```python
from build123d import *

# Parameters (mm, degrees)
BOSS_EXTRUDE1_DEPTH = 3
SKETCH2_R           = 1.5
CUT_EXTRUDE1_DEPTH  = 302.770194022
SKETCH3_R           = 1.5
CUT_EXTRUDE2_DEPTH  = 302.770194022
LPATTERN1_COUNT     = 6
LPATTERN1_PITCH     = 15


with BuildPart() as part:
    # Sketch1 → Boss-Extrude1 (new body)
    with BuildSketch(Plane(origin=(0, 0, 0), x_dir=(1, 0, 0), z_dir=(0, 1, 0))):
        Polygon((32.5, 300), (-32.5, 300), (-32.5, 270), (-15, 270), (-15, 90), (-21, 90), (-21, 0), (21, 0), (21, 90), (15, 90), (15, 270), (32.5, 270), align=None)
    extrude(amount=BOSS_EXTRUDE1_DEPTH)

    # Sketch2 → Cut-Extrude1 (cut, symmetric)
    with BuildSketch(Plane(origin=(0, 3, 0), x_dir=(1, 0, 0), z_dir=(0, 1, 0))):
        with Locations(Location((-28, 295.85, 0), (0, 0, 270))):
            Circle(SKETCH2_R)
        with Locations(Location((-7, 295.85, 0), (0, 0, 270))):
            Circle(SKETCH2_R)
        with Locations(Location((-28, 274.15, 0), (0, 0, 270))):
            Circle(SKETCH2_R)
        with Locations(Location((-7, 274.15, 0), (0, 0, 270))):
            Circle(SKETCH2_R)
    cut_extrude1 = extrude(amount=CUT_EXTRUDE1_DEPTH, both=True, mode=Mode.SUBTRACT)

    # Mirror1: Cut-Extrude1 across plane
    add(cut_extrude1.mirror(Plane(origin=(0, 0, 0), x_dir=(0, 0, 1), z_dir=(1, 0, 0))), mode=Mode.SUBTRACT)

    # Sketch3 → Cut-Extrude2 (cut, symmetric)
    with BuildSketch(Plane(origin=(0, 3, 0), x_dir=(1, 0, 0), z_dir=(0, 1, 0))):
        with BuildLine():
            ThreePointArc((-11, 82), (-11.439339828, 83.060660172), (-12.5, 83.5))
            Line((-12.5, 83.5), (-12.5, 80.5))
            ThreePointArc((-12.5, 80.5), (-11.439339828, 80.939339828), (-11, 82))
        make_face()
        with BuildLine():
            Line((-12.5, 80.5), (-12.5, 83.5))
            ThreePointArc((-12.5, 83.5), (-14, 82), (-12.5, 80.5))
        make_face()
        with Locations(Location((12.5, 82, 0), (0, 0, 270))):
            Circle(SKETCH3_R)
    cut_extrude2 = extrude(amount=CUT_EXTRUDE2_DEPTH, both=True, mode=Mode.SUBTRACT)

    # LPattern1: Cut-Extrude2 ×6
    with Locations(*[(0, 0, i * LPATTERN1_PITCH) for i in range(1, LPATTERN1_COUNT)]):
        add(cut_extrude2, mode=Mode.SUBTRACT)


solid = part.part
```
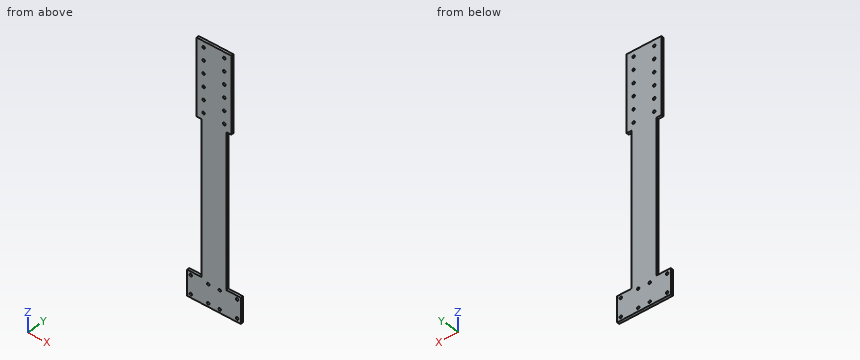
Here's how the part is built. I have some questions about the finished solid (model axes, mm). Give positions to 0.01 mm unless a question says otherwise; leave off trailing zeros. Write each loop counter-clockwise with the first axis right and the second up, starting at its lowest first coordinate (ties: lowest second). Pieces come first, ordered by that corner, then holes. Notation, with made-up numbers: (15, -17) -> (50, -17) arc R19 cw to (50, -13) -> close; hole circle Ø3 at (-20.75, 39). An arc over 180 degrees is marked (long way). Write each question's results on one line, items separated by ' | '.
Item 1: For pin 1 Ø4 at (x, z) = (-28, -295.85) entering from -Y; pin 2 Ø1.5 at (x, y) = (-27, 1) entering from +Z; pin 3 Ø0.9 at (y, z) = (2, -29) entering from +X, each with a flat end and sliding along its axis, tell me the tip position at first contact or that it passes through.
Output:
pin 1: stops at y = 0 | pin 2: stops at z = -270 | pin 3: stops at x = 21
Item 2: Suppose I cut it at A-A on y = 1.85. Give the number of separate pieces and of enclosed holes in the cut face, plus the area to 3 significant figures.
Output:
separate pieces: 1 | enclosed holes: 20 | area: 11,000 mm^2
Item 3: If I drill on L1, parallel to Z at x = 28, y = 1.55; L2, parallel to X at y = 2.3, z = -274.15; L3, parallel to Z at x = -15.5, y = 1.3, over which ranges is the centre line in solid material (lowest first)?
Output:
L1: z = -300 to -297.35, -294.35 to -275.65, -272.65 to -270 | L2: x = -32.5 to -29.5, -26.5 to -8.5, -5.5 to 5.5, 8.5 to 26.5, 29.5 to 32.5 | L3: z = -300 to -270, -90 to 0
Item 4: Suppose I cut it at C-C on z = -61. Write out the boundary of the cut face in (x, y), plus the area to 3 significant figures.
Output:
outline: (-21, 0) -> (21, 0) -> (21, 3) -> (-21, 3) -> close | area: 126 mm^2
Item 5: Suppose I cut it at B-B on z = -103. Write out the boundary of the cut face in (x, y), plus the area to 3 significant figures.
Output:
outline: (-15, 0) -> (15, 0) -> (15, 3) -> (-15, 3) -> close | area: 90.0 mm^2
